from build123d import *

# Parameters (mm, degrees)
CROQUIS1_R              = 26
CROQUIS1_R_2            = 2
SALIENTE_EXTRUIR1_DEPTH = 2.5
REDONDEO1_R             = 1


with BuildPart() as part:
    # Croquis1 → Saliente-Extruir1 (new body)
    with BuildSketch(Plane(origin=(0, 0, 0), x_dir=(1, 0, 0), z_dir=(0, 1, 0))):
        with BuildLine():
            Line((-32, 6), (-31.432467291, 6))
            ThreePointArc((-31.432467291, 6), (0, 32), (31.432467291, 6))
            Line((31.432467291, 6), (32, 6))
            ThreePointArc((32, 6), (38, 0), (32, -6))
            Line((32, -6), (31.432467291, -6))
            ThreePointArc((31.432467291, -6), (0, -32), (-31.432467291, -6))
            Line((-31.432467291, -6), (-32, -6))
            ThreePointArc((-32, -6), (-38, 0), (-32, 6))
        make_face()
        with Locations(Location((0, 0, 0), (0, 0, 270))):
            Circle(CROQUIS1_R, mode=Mode.SUBTRACT)
        with Locations(Location((-32, 0, 0), (0, 0, 270))):
            Circle(CROQUIS1_R_2, mode=Mode.SUBTRACT)
        with Locations(Location((32, 0, 0), (0, 0, 270))):
            Circle(CROQUIS1_R_2, mode=Mode.SUBTRACT)
    extrude(amount=SALIENTE_EXTRUIR1_DEPTH)

    # Redondeo1
    redondeo1_edges = [part.edges().sort_by_distance(p)[0] for p in [
        (0, 2.5, -32),
        (-31.716233646, 2.5, -6),
        (-38, 2.5, 0),
        (0, 2.5, -26),
        (-31.716233646, 2.5, 6),
        (0, 2.5, 32),
        (31.716233646, 2.5, 6),
        (38, 2.5, 0),
        (31.716233646, 2.5, -6),
    ]]
    fillet(redondeo1_edges, radius=REDONDEO1_R)


solid = part.part
Read the model definition and answer for the solid it produces. Units are mm, in the model's axes. Round coordinates to 2 decimals unless told otherwise and drop trailing zeros. Order: outer loops, then holes, each group sorted by start corner. A loop starts at its lowest first (then second) coordinate and runs counter-clockwise, first axis right, second up.
1) The mould has two halves that part along X. Classify faces 1 (the face through (-0.619, 0.74, -31.994)), 2 (the face through (-15.821, 0.74, -20.633)), 3 (the face through (38, 1, 0)), 4 (the face through (30, 1, 0)): released by +X, released by -X, zero draft, split by the parting line, or undercut.
2) The part is cut by section B-B on y = 0.9. Write down the section's boundary in (x, z), plus the area to 3 significant figures.
3) The part is cut by section C-C on z = -1. Give the number of separate pieces and of enclosed holes in the cut face, plus the area to 3 significant figures.
4) Flat-ended cylindrical pins translate along their axes: pin 1 (3 mm diameter, centred on x = -32, z = 0, fed in from -Y); pin 2 (0.6 mm diameter, centred on x = 32, y = 1, fed in from +Z). Find the tip coordinate at first contact, or state that the pin passes through.
5) The part is cut by section A-A on x = 0. Write down the section's boundary in (y, z).
6) Straight lines are drawn through the part: L1, parallel to X at y = 1.15, z = 0; L2, parallel to Z at x = -5.5, y = 1.9; L3, parallel to Z at x = -24, y = 0.9. For each, find the intervals that lie inside material, in ascending order.
Resolved:
1. face 1: split by the parting line
1. face 2: undercut
1. face 3: released by +X
1. face 4: undercut
2. outline: (-32, -6) - (-31.43, -6) arc R32 ccw to (31.43, -6) - (32, -6) arc R6 ccw to (32, 6) - (31.43, 6) arc R32 ccw to (-31.43, 6) - (-32, 6) arc R6 ccw to start; hole circle Ø4 at (-32, 0); hole circle Ø52 at (0, 0); hole circle Ø4 at (32, 0)
2. area: 1,190 mm2
3. separate pieces: 4
3. enclosed holes: 0
3. area: 41.5 mm2
4. pin 1: passes through
4. pin 2: stops at z = 6
5. outline: (0, -32) - (1.5, -32) arc R1 ccw to (2.5, -31) - (2.5, -27) arc R1 ccw to (1.5, -26) - (0, -26) - close; (0, 26) - (1.5, 26) arc R1 ccw to (2.5, 27) - (2.5, 31) arc R1 ccw to (1.5, 32) - (0, 32) - close
6. L1: x = -38 to -34, -30 to -26, 26 to 30, 34 to 38
6. L2: z = -31.44 to -25.5, 25.5 to 31.44
6. L3: z = -21.17 to -10, 10 to 21.17
